from build123d import *

# Parameters (mm, degrees)
F0_W     = 40
F0_H     = 30
F1_DEPTH = 12.5
F2_R     = 5
F3_DEPTH = 58


with BuildPart() as f1:
    # F0 (on Front) → F1 (new body, symmetric)
    with BuildSketch(Plane.XZ):
        Rectangle(F0_W, F0_H)
    extrude(amount=F1_DEPTH, both=True)

    # F2 (on face) → F3 (cut)
    with BuildSketch(Plane.YZ.offset(20)):
        Circle(F2_R)
    extrude(amount=-F3_DEPTH, mode=Mode.SUBTRACT)


solid = f1.part
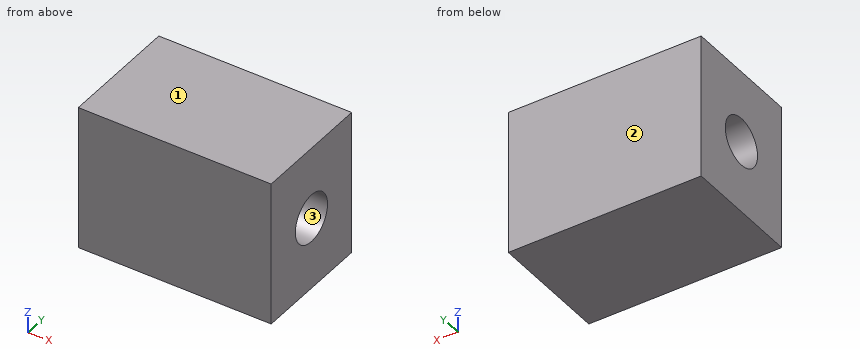
Design review of the part built by this model. Coordinates are the model's own, in mm. Face numbers are marked on the shaded views. Coordinates: 2 decimals unless noted, no trailing zeros. Order: outer loops, then holes, each group sorted by start corner. A loop starts at its lowest first (then second) coordinate and runs counter-clockwise, first axis right, second up. Notation, with made-up numbers: M 72.5,87.25 L 95.5,87.25 A18 ccw 95.5,116.25 Z; hole C -23,3.5 d2. An arc over 180 degrees is marked long. Use a Markdown table: item, result.
(1) Add section C-C (x = -1). Give the boundary of the cut face in (y, z), then the cut area to 3 significant figures.
Worked answers:
| item | result |
|---|---|
| outline | M -12.5,-15 L 12.5,-15 L 12.5,15 L -12.5,15 Z; hole C 0,0 d10 |
| area | 671 mm2 |
(2) Add section A-A (y = 0). Give the boundary of the cut face in (x, z).
Worked answers:
| item | result |
|---|---|
| outline | M -20,-15 L 20,-15 L 20,-5 L -20,-5 Z; M -20,5 L 20,5 L 20,15 L -20,15 Z |
(3) Draft analysis for pull direction Y (two halves, no side actions). For the marked faces 1, 2 and 3, state which applies: released by +Y, released by -Y, zero draft, split by the parting line, or undercut.
Worked answers:
| item | result |
|---|---|
| face 1 | zero draft |
| face 2 | released by +Y |
| face 3 | undercut |
(4) Add section B-B (z = 0). Give the boundary of the cut face in (x, y), then the cut area to 3 significant figures.
Worked answers:
| item | result |
|---|---|
| outline | M -20,-12.5 L 20,-12.5 L 20,-5 L -20,-5 Z; M -20,5 L 20,5 L 20,12.5 L -20,12.5 Z |
| area | 600 mm2 |
(5) Wall thickness on probe 1 along Z at (x, y) = (8.5, 0); probe 2 along Y at (x, z) = (-8, 1.25); probe 3 along Y at (x, z) = (9, 3): over which ranges is each line inside the solid? List them lowest first.
Worked answers:
| item | result |
|---|---|
| probe 1 | z = -15 to -5, 5 to 15 |
| probe 2 | y = -12.5 to -4.84, 4.84 to 12.5 |
| probe 3 | y = -12.5 to -4, 4 to 12.5 |
